Geometry: final body of the model. Coordinates: model frame, mm. A direction names the side the tool comes from. Coordinates: 2 decimals unless noted, no trailing zeros. Write each loop counter-clockwise with the first axis right and the second up, starting at its lowest first coordinate (ties: lowest second). Pieces come first, ordered by that corner, then holes.
from build123d import *

# Parameters (mm, degrees)
SKETCH2_W           = 30
SKETCH2_H           = 30
BOSS_EXTRUDE2_DEPTH = 30
SKETCH4_W           = 6
SKETCH4_H           = 30
BOSS_EXTRUDE3_DEPTH = 30
FILLET4_R           = 10
SKETCH5_R           = 6
CUT_EXTRUDE1_DEPTH  = 30
FILLET5_R           = 6
SKETCH6_R           = 6.1
CUT_EXTRUDE2_DEPTH  = 62
FILLET6_R           = 6


with BuildPart() as part:
    # Sketch2 → Boss-Extrude2 (new body)
    with BuildSketch(Plane.XY):
        Rectangle(SKETCH2_W, SKETCH2_H)
    extrude(amount=BOSS_EXTRUDE2_DEPTH)

    # Sketch4 → Boss-Extrude3 (add)
    with BuildSketch(Plane(origin=(0, 15, 0), x_dir=(1, 0, 0), z_dir=(0, 1, 0))):
        with Locations((-12, -15)):
            Rectangle(SKETCH4_W, SKETCH4_H)
        with Locations((12, -15)):
            Rectangle(SKETCH4_W, SKETCH4_H)
    extrude(amount=BOSS_EXTRUDE3_DEPTH)

    # Fillet4
    fillet4_edges = [part.edges().sort_by_distance(p)[0] for p in [
        (-12, 45, 30),
        (-12, 45, 0),
        (12, 45, 30),
        (12, 45, 0),
    ]]
    fillet(fillet4_edges, radius=FILLET4_R)

    # Sketch5 → Cut-Extrude1 (cut)
    with BuildSketch(Plane.ZY.offset(15)):
        with Locations(Location((15, 35, 0), (0, 0, 270))):
            Circle(SKETCH5_R)
    extrude(amount=-CUT_EXTRUDE1_DEPTH, mode=Mode.SUBTRACT)

    # Fillet5
    fillet5_edges = [part.edges().sort_by_distance(p)[0] for p in [
        (-9, 15, 15),
        (9, 15, 15),
    ]]
    fillet(fillet5_edges, radius=FILLET5_R)

    # Sketch6 → Cut-Extrude2 (cut)
    with BuildSketch(Plane.ZY.offset(15)):
        with Locations(Location((15, 2.384259025, 0), (0, 0, 270))):
            Circle(SKETCH6_R)
    extrude(amount=-CUT_EXTRUDE2_DEPTH, mode=Mode.SUBTRACT)

    # Fillet6
    fillet6_edges = [part.edges().sort_by_distance(p)[0] for p in [
        (0, -15, 30),
        (0, -15, 0),
    ]]
    fillet(fillet6_edges, radius=FILLET6_R)


solid = part.part
Item 1: Set-up query: faces 1 (the cylindrical face through (7.196, 16.711, 14.79)), 2 (the cylindrical face through (12, 41, 15)). Return all of +Z, -Z, +X, -X, +Y, -Y with unobstructed straight access to the full face (end or side cutting, diameter ignored); none if empty.
Derived:
face 1: +Z, -Z, +Y
face 2: +X, -X
Item 2: Section A-A, the plane y = 28. Output: boundary loops of the cut face in (x, z).
Derived:
outline: (-15, 0) - (-9, 0) - (-9, 30) - (-15, 30) - close; (9, 0) - (15, 0) - (15, 30) - (9, 30) - close
Item 3: Material intervals for probe 1 along Z at (x, y) = (13.05, 35); probe 2 along X at (y, z) = (29, 3.25); probe 3 along Y at (x, z) = (13.5, 12.5), sorted ascending.
Derived:
probe 1: z = 0 to 9, 21 to 30
probe 2: x = -15 to -9, 9 to 15
probe 3: y = -15 to -3.18, 7.95 to 29.55, 40.45 to 45
Item 4: Section D-D, the plane z = 22.5. Output: boundary loops of the cut face in (x, y), plus the area to 3 significant figures.
Derived:
outline: (-15, -15) - (15, -15) - (15, 44.68) - (9, 44.68) - (9, 21) arc R6 cw to (3, 15) - (-3, 15) arc R6 cw to (-9, 21) - (-9, 44.68) - (-15, 44.68) - close
area: 1,270 mm2
Item 5: Pin query (flat end, axial travel): pin 1 (11 mm diameter, centred on y = 2.38, z = 15, fed in from +X); pin 2 (6.5 mm diameter, centred on x = 1, z = 22.5, fed in from +Y). Return the tip coordinate at first contact, or that it passes through.
Derived:
pin 1: passes through
pin 2: stops at y = 15.13
Item 6: Section C-C, the plane x = 10.75. Output: boundary loops of the cut face in (y, z).
Derived:
outline: (-15, 6) arc R6 ccw to (-9, 0) - (35, 0) arc R10 ccw to (45, 10) - (45, 20) arc R10 ccw to (35, 30) - (-9, 30) arc R6 ccw to (-15, 24) - close; hole circle Ø12.2 at (2.38, 15); hole circle Ø12 at (35, 15)
Item 7: Section B-B, the plane x = -1.75. Output: boundary loops of the cut face in (y, z).
Derived:
outline: (-15, 6) arc R6 ccw to (-9, 0) - (15, 0) - (15, 30) - (-9, 30) arc R6 ccw to (-15, 24) - close; hole circle Ø12.2 at (2.38, 15)
Item 8: Pull-direction query (X, two-part tool) for faces 3 (the flat face through (9, 27, 15)), 4 (the flat face through (-15, 15, 15)), 5 (the flat face through (12, 45, 15)); classes: released by +X, released by -X, zero draft, split by the parting line, or undercut.
Derived:
face 3: undercut
face 4: released by -X
face 5: zero draft
